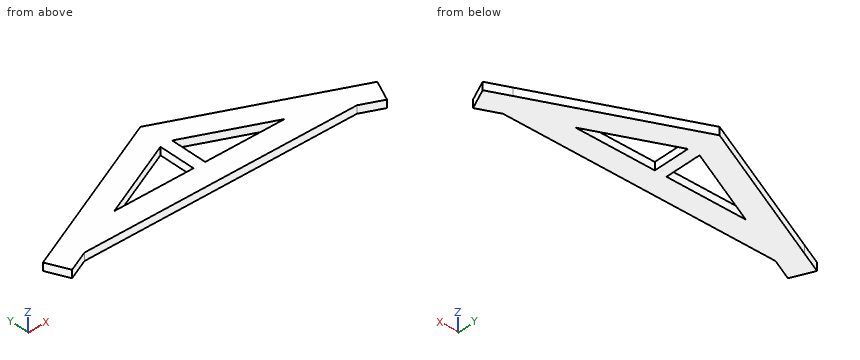
from build123d import *

# Parameters (mm, degrees)
F1_DEPTH = 2


with BuildPart() as f1:
    # F0 (on Top) → F1 (new body)
    with BuildSketch(Plane.XY):
        Polygon((-35, 0), (0, 0), (35, 0), (40.456847, -2.494559), (42.951405, 2.962288), (37.494559, 5.456847), (0, 22.597216), (-37.494559, 5.456847), (-42.951405, 2.962288), (-40.456847, -2.494559), align=None)
        Polygon((-21.875, 6), (-1.5, 15.314286), (-1.5, 6), align=None, mode=Mode.SUBTRACT)
        Polygon((1.5, 6), (1.5, 15.314286), (21.875, 6), align=None, mode=Mode.SUBTRACT)
    extrude(amount=F1_DEPTH)


solid = f1.part
The listing builds one solid part. Answer for the finished solid, in the listing's coordinates (mm). Give positions to 0.01 mm unless a question says otherwise; leave off trailing zeros. Loops run counter-clockwise (first coordinate to the right, second up) from the corner with the lowest first, then second, coordinate; pieces in that order, holes last. Notation, with made-up numbers: (14.25, 24) - (54.25, 24) arc R31 cw to (54.25, 59) - close; hole circle Ø10 at (72.5, 55). An arc over 180 degrees is marked (long way). Use one line per item in the form item = value.
1. Given pin 1 Ø1 at (y, z) = (3.5, 1) entering from -X; pin 2 Ø0.6 at (y, z) = (12, 1) entering from +X; pin 3 Ø1 at (y, z) = (0.5, 1) entering from +X, each flat-ended and moving along its own axis, determine where each tip first touches the part or whether it passes through.
Calculated:
pin_1 = -42.87
pin_2 = 23.84
pin_3 = 42.05
2. Find the intervals of material crossed by line 1 along X through (y, z) = (12, 1.65); line 2 along X through (y, z) = (6.5, 1.3); line 3 along Y through (x, z) = (-5.5, 1), in increasing order. Write a range as [from, to].
Calculated:
line_1 = [-23.18, -8.75], [-1.5, 1.5], [8.75, 23.18]
line_2 = [-35.21, -20.78], [-1.5, 1.5], [20.78, 35.21]
line_3 = [0, 6], [13.49, 20.08]
3. Section A-A on z = 1.15 is taken. Give the vertices of the cut face in (x, y) (3 decimals).
Calculated:
outline = (-42.951, 2.962) - (-40.457, -2.495) - (-35, 0) - (35, 0) - (40.457, -2.495) - (42.951, 2.962) - (37.495, 5.457) - (0, 22.597) - (-37.495, 5.457) - close; hole (-21.875, 6) - (-1.5, 6) - (-1.5, 15.314) - close; hole (1.5, 6) - (21.875, 6) - (1.5, 15.314) - close
4. Section B-B on y = 7.5 is taken. Give the vertices of the cut face in (x, z), then the cut area to 3 significant figures.
Calculated:
outline = (-33.03, 0) - (-18.59, 0) - (-18.59, 2) - (-33.03, 2) - close; (-1.5, 0) - (1.5, 0) - (1.5, 2) - (-1.5, 2) - close; (18.59, 0) - (33.03, 0) - (33.03, 2) - (18.59, 2) - close
area = 63.7 mm^2
5. Section C-C on x = -14 is taken. Give the vertices of the cut face in (y, z).
Calculated:
outline = (0, 0) - (6, 0) - (6, 2) - (0, 2) - close; (9.6, 0) - (16.2, 0) - (16.2, 2) - (9.6, 2) - close
6. Section D-D on y = 19 is taken. Give the vertices of the cut face in (x, z).
Calculated:
outline = (-7.87, 0) - (7.87, 0) - (7.87, 2) - (-7.87, 2) - close
